Autodesk Fusion 360 part; units mm, degrees
sketch "Sketch1" plane through (0, 0, 0) normal (0, 0, 1) x (1, 0, 0)
  line L0 (-74, -11) -> (-16, -11)
  line L1 (-16, 11) -> (-74, 11)
  arc A0 (-74, 11) -> (-74, -11) centre (-74, 0) ccw
  arc A1 (-16, -11) -> (-16, 11) centre (-16, 0) ccw
  circle A2 centre (-74, 0) radius 2
  circle A3 centre (-16, 0) radius 2
  line L2 (-63, 11) -> (-63, -11)
  line L3 (-27, 11) -> (-27, -11)
  line L4 (-63, 7) -> (-27, 7)
  line L5 (-63, -7) -> (-27, -7)
  dimension "d1" = 4
  dimension "d2" = 4
extrude "Extrude1" add sketch "Sketch1" along normal blind 12 contours L0 L1 A0 L2 | L0 L1 A1 L3 makes body 1 at (-66, 0, 0) makes body 2 at (-24, 0, 0)
extrude "Extrude2" add sketch "Sketch1" along normal blind 6 contours L2 L3 L4 L5 bodies 1 2
chamfer "Chamfer1" distance 1.5 angle 45 2 edges at (-75.8647, 0.7232, 0) (-17.8647, 0.7232, 0) on bodies 1
fillet "Fillet1" radius 2 4 edges at (-63, -7, 3) (-27, -7, 3) (-27, 7, 3) (-63, 7, 3) on bodies 1
fillet "Fillet2" radius 2 4 edges at (-63, 11, 6) (-27, 11, 6) (-27, -11, 6) (-63, -11, 6) on bodies 1
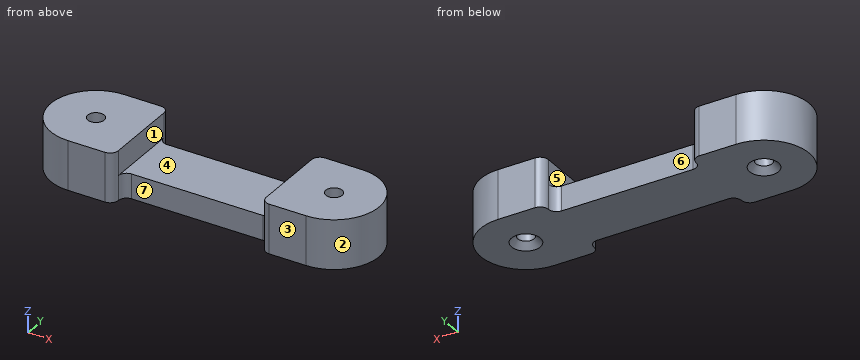
Here's how the part is built. I have some questions about the finished solid (model axes, mm). Face numbers are marked on the shaded views. A direction names the side the tool comes from. Coordinates: 2 decimals unless noted, no trailing zeros. Order: outer loops, then holes, each group sorted by start corner. A loop starts at its lowest first (then second) coordinate and runs counter-clockwise, first axis right, second up. Notation, with made-up numbers: M 61.25,-33.75 L 80.25,-33.75 A9 cw 80.25,-22.75 Z; hole C 32.5,2 d7. An arc over 180 degrees is marked long. Answer as a JSON object with one key per item and string values. Group by question number.
(1) For pin 1 (2 mm diameter, centred on x = -72.5, y = -0.5, fed in from +Z); pin 2 (5 mm diameter, centred on y = -3, z = 9.5, fed in from +X); pin 3 (1.8 mm diameter, centred on x = -47.5, z = 3.5, fed in from -Y); pin 4 (1.8 mm diameter, centred on x = -44.5, z = 4, fed in from +Y), each with a flat end and sliding along its axis, tell me the tip position at first contact or that it passes through.
(2) I need wall thicknesses on probe 1 along Y at (x, z) = (-16, 9.5); probe 2 along X at (y, z) = (0.5, 10.75); probe 3 along X at (y, z) = (5, 6.25). Which ranges of each line are inside material? Lowest first, please.
(3) Suppose I cut it at C-C, the plane z = 3.5. Please give me the cut outline in (x, y), then the cut area to 3 significant figures.
(4) Suppose I cut it at A-A, the plane z = 8. Please give me the cut outline in (x, y).
(5) Which directions (+Z, -Z, +X, -X, +Y, -Y) give clear straight access to the entire face, cutting with the end or side of a thin tool? Please do the marked faces 5, 6 and 7.
(6) Suppose I cut it at D-D, the plane y = 8. Please give me the cut outline in (x, z), then the cut area to 3 significant figures.
(7) If we mould it in two halves opening along X, with no side actions, what happens to the marked faces 1, 2, 3 and 4? For each: released by +X, released by -X, zero draft, split by the parting line, or undercut.
(8) Suppose I cut it at B-B, the plane y = 0. Please give me the cut outline in (x, z), then the cut area to 4 significant figures.
Values found:
{
 "1": {"pin 1": "stops at z = 12", "pin 2": "stops at x = -5.01", "pin 3": "stops at y = -7", "pin 4": "stops at y = 7"},
 "2": {"probe 1": "y = -11 to -2, 2 to 11", "probe 2": "x = -84.99 to -75.94, -72.06 to -63, -27 to -17.94, -14.06 to -5.01", "probe 3": "x = -83.8 to -63, -27 to -6.2"},
 "3": {"outline": "M -74,-11 L -65,-11 A2 ccw -63,-9 A2 cw -61,-7 L -29,-7 A2 cw -27,-9 A2 ccw -25,-11 L -16,-11 A11 ccw -16,11 L -25,11 A2 ccw -27,9 A2 cw -29,7 L -61,7 A2 cw -63,9 A2 ccw -65,11 L -74,11 A11 ccw Z; hole C -74,0 d4; hole C -16,0 d4", "area": "1,340 mm^2"},
 "4": {"outline": "M -74,-11 L -65,-11 A2 ccw -63,-9 L -63,9 A2 ccw -65,11 L -74,11 A11 ccw Z; M -27,-9 A2 ccw -25,-11 L -16,-11 A11 ccw -16,11 L -25,11 A2 ccw -27,9 Z; hole C -74,0 d4; hole C -16,0 d4"},
 "5": {"face 5": "+Z, +Y, -Y", "face 6": "+Z, -Z, +Y", "face 7": "+Z, -Z, -Y"},
 "6": {"outline": "M -81.55,0 L -62.73,0 L -62.73,6 L -63,6 L -63,12 L -81.55,12 Z; M -27.27,0 L -8.45,0 L -8.45,12 L -27,12 L -27,6 L -27.27,6 Z", "area": "448 mm^2"},
 "7": {"face 1": "undercut", "face 2": "released by +X", "face 3": "zero draft", "face 4": "undercut"},
 "8": {"outline": "M -85,0 L -77.5,0 L -76,1.5 L -76,12 L -85,12 Z; M -72,1.5 L -70.5,0 L -19.5,0 L -18,1.5 L -18,12 L -27,12 L -27,6 L -63,6 L -63,12 L -72,12 Z; M -14,1.5 L -12.5,0 L -5,0 L -5,12 L -14,12 Z", "area": "643.5 mm^2"}
}
